Could you check a few things on this model? Use its own coordinates, in mm. A direction names the side the tool comes from. Coordinates: 2 decimals unless noted, no trailing zeros. Order: outer loops, then holes, each group sorted by start corner. A loop starts at its lowest first (then second) coordinate and runs counter-clockwise, first axis right, second up. Notation, with made-up numbers: (-10, 36.25) -> (-4, 36.25) arc R22 cw to (-4, 58.25) -> close; hole circle Ø2 at (37.25, 39). An arc over 180 degrees is marked (long way). Put each result on its own line as item: value. Start each with the question number.
Q1. Will these pins go through, and if not, where does the flat tip stop? pin 1 (10 mm diameter, centred on x = -25, y = -12, fed in from +Z); pin 2 (8 mm diameter, centred on x = 40.95, z = -32.32, fed in from +Y); pin 3 (1 mm diameter, centred on x = -19.5, z = 14, fed in from +Y); pin 4 (12 mm diameter, centred on x = 0, z = 0, fed in from -Y).
Q2. If we section it at C-C (x = 48): Please give me the cut outline in (y, z), and give its area (3 significant figures).
Q3. If we section it at B-B (y = 17): Please give me the cut outline in (x, z), and give its area (3 significant figures).
Q4. Please list where these lines run through material, in increasing order: line 1 along X through (y, z) = (21, 29.5); line 2 along Z through (x, y) = (35, 9); line 3 along Z through (x, y) = (37.5, 5.5).
Q5. We'd pull the mould along Z, two halves only. Please class faces 6 (the face through (-52.7, 15, 1)), 7 (the face through (-50.7, 15, 1)), 8 (the face through (-1, 15, -42.7)): +Z half, -Z half, draft (parallel to the pull), parting line (faces both ways), or undercut.
Q6. If we section it at A-A (y = 10): Count the separate pieces of the cut face and the enclosed holes in it, and give its area (3 significant figures).
Q7. For faces 1 (the face through (-1, 15, -40.7)), 2 (the face through (33.71, -12.32, 4.43)), 3 (the face through (-1, 15, 42.7)), 4 (the face through (-1, 2, -45)), 5 (the face through (-51, 25, 0)), which set-ups out of +Z, -Z, +X, -X, +Y, -Y let a thin tool reach every point of the face, with its end or its side?
from build123d import *

# Parameters (mm, degrees)
SKETCH1_W           = 110
SKETCH1_H           = 90
BOSS_EXTRUDE1_DEPTH = 5
SKETCH4_W           = 105.4
SKETCH4_H           = 85.4
SKETCH4_W_2         = 101.4
SKETCH4_H_2         = 81.4
BOSS_EXTRUDE2_DEPTH = 20
SKETCH5_R           = 5
BOSS_EXTRUDE3_DEPTH = 7
SKETCH9_R           = 2.524761235
CUT_EXTRUDE1_DEPTH  = 5
SKETCH10_R          = 34
BOSS_EXTRUDE4_DEPTH = 25
SKETCH11_R          = 10.080259213
CUT_EXTRUDE2_DEPTH  = 31
CUT_EXTRUDE3_DEPTH  = 23


with BuildPart() as part:
    # Sketch1 → Boss-Extrude1 (new body)
    with BuildSketch(Plane(origin=(0, 0, 0), x_dir=(1, 0, 0), z_dir=(0, 1, 0))):
        Rectangle(SKETCH1_W, SKETCH1_H)
    extrude(amount=BOSS_EXTRUDE1_DEPTH)

    # Sketch4 → Boss-Extrude2 (add)
    with BuildSketch(Plane(origin=(0, 5, 0), x_dir=(1, 0, 0), z_dir=(0, 1, 0))):
        Rectangle(SKETCH4_W, SKETCH4_H)
        Rectangle(SKETCH4_W_2, SKETCH4_H_2, mode=Mode.SUBTRACT)
    extrude(amount=BOSS_EXTRUDE2_DEPTH)

    # Sketch5 → Boss-Extrude3 (add)
    with BuildSketch(Plane(origin=(0, 5, 0), x_dir=(1, 0, 0), z_dir=(0, 1, 0))):
        with Locations(Location((-40.846907762, 32.318983418, 0), (0, 0, 270))):
            Circle(SKETCH5_R)
        with Locations(Location((-40.846907762, -31.281016582, 0), (0, 0, 270))):
            Circle(SKETCH5_R)
        with Locations(Location((40.953092238, -31.273370815, 0), (0, 0, 270))):
            Circle(SKETCH5_R)
        with Locations(Location((40.953092238, 32.318983418, 0), (0, 0, 270))):
            Circle(SKETCH5_R)
    extrude(amount=BOSS_EXTRUDE3_DEPTH)

    # Sketch9 → Cut-Extrude1 (cut)
    with BuildSketch(Plane(origin=(0, 12, 0), x_dir=(1, 0, 0), z_dir=(0, 1, 0))):
        with Locations(Location((40.953092238, 32.318983418, 0), (0, 0, 270))):
            Circle(SKETCH9_R)
        with Locations(Location((40.953092238, -31.273370815, 0), (0, 0, 270))):
            Circle(SKETCH9_R)
        with Locations(Location((-40.846907762, -31.273370815, 0), (0, 0, 270))):
            Circle(SKETCH9_R)
        with Locations(Location((-40.846907762, 32.318983418, 0), (0, 0, 270))):
            Circle(SKETCH9_R)
    extrude(amount=-CUT_EXTRUDE1_DEPTH, mode=Mode.SUBTRACT)

    # Sketch10 → Boss-Extrude4 (add)
    with BuildSketch(Plane.XZ):
        with Locations(Location((0, 0, 0), (0, 0, 270))):
            Circle(SKETCH10_R)
    extrude(amount=BOSS_EXTRUDE4_DEPTH)

    # Sketch11 → Cut-Extrude2 (cut)
    with BuildSketch(Plane(origin=(0, -25, 0), x_dir=(-1, 0, 0), z_dir=(0, -1, 0))):
        with Locations(Location((0, 0, 0), (0, 0, 90))):
            Circle(SKETCH11_R)
    extrude(amount=-CUT_EXTRUDE2_DEPTH, mode=Mode.SUBTRACT)

    # 3DSketch1 → Cut-Extrude3 (cut)
    with BuildSketch(Plane(origin=(0, -25, -32), x_dir=(-0.004227803372085143, 0, 0.9999910627993868), z_dir=(0, 1, 0))):
        with BuildLine():
            add(Edge.make_bspline(
                [(0, 0), (-0.011789907, 2.799656794), (0.703810307, 8.402918744), (3.921124481, 16.240807355), (9.062436479, 22.975250557), (15.774929183, 28.145163081), (23.599222448, 31.395708592), (31.998932575, 32.504978995), (40.398695895, 31.396113621), (48.223147077, 28.145948653), (54.935885594, 22.976350086), (60.077545593, 16.242187891), (63.295168912, 8.404298627), (64.369120742, 0), (63.224955208, -8.395027888), (59.941927667, -16.205747313), (54.744156701, -22.896695338), (47.988440156, -28.01000158), (40.137094558, -31.194649365), (31.728354863, -32.233260194), (23.338213795, -31.053824953), (15.541353588, -27.737955266), (8.872355042, -22.512245002), (3.841180978, -15.806348738), (0.727018017, -8.127446073), (0.01141332, -2.710231546), (0, 0)],
                knots=[0, 0, 0, 0, 0.041777734, 0.083555145, 0.125332704, 0.167110267, 0.208887828, 0.25066539, 0.292442951, 0.334220512, 0.375998074, 0.417775635, 0.459553197, 0.501330758, 0.543108319, 0.584885881, 0.626663442, 0.668441003, 0.710218565, 0.751996126, 0.793773688, 0.835551249, 0.877328803, 0.919106374, 0.95955671, 1, 1, 1, 1], degree=3))
        make_face()
    extrude(amount=CUT_EXTRUDE3_DEPTH, mode=Mode.SUBTRACT)


solid = part.part
The answers:
1. pin 1: z = 27.5
1. pin 2: y = 12
1. pin 3: y = 5
1. pin 4: through
2. outline: (0, -45) -> (5, -45) -> (5, -42.7) -> (25, -42.7) -> (25, -40.7) -> (5, -40.7) -> (5, 40.7) -> (25, 40.7) -> (25, 42.7) -> (5, 42.7) -> (5, 45) -> (0, 45) -> close
2. area: 530 mm^2
3. outline: (-52.7, -42.7) -> (52.7, -42.7) -> (52.7, 42.7) -> (-52.7, 42.7) -> close; hole (-50.7, -40.7) -> (50.7, -40.7) -> (50.7, 40.7) -> (-50.7, 40.7) -> close
3. area: 747 mm^2
4. line 1: -52.7 to -50.7, 50.7 to 52.7
4. line 2: -42.7 to -40.7, 40.7 to 42.7
4. line 3: -42.7 to -40.7, -35.94 to -28.7, 27.66 to 34.89, 40.7 to 42.7
5. face 6: draft
5. face 7: undercut
5. face 8: -Z half
6. separate pieces: 5
6. enclosed holes: 5
6. area: 981 mm^2
7. face 1: +Y
7. face 2: -Y
7. face 3: +Z, +X, -X, +Y
7. face 4: -Z, +X, -X, +Y, -Y
7. face 5: +Z, -Z, +X, -X, +Y
